Autodesk Inventor part; units mm, degrees
ref_plane "YZ Plane" through (0, 0, 0) normal (1, 0, 0) x (0, 1, 0)
ref_plane "XZ Plane" through (0, 0, 0) normal (0, 1, 0) x (-1, 0, 0)
ref_plane "XY Plane" through (0, 0, 0) normal (0, 0, 1) x (1, 0, 0)
sketch "Sketch1" plane through (0, 0, 0) normal (0, 0, 1) x (1, 0, 0)
  line L0 (-73, -33) -> (73, -33)
  line L1 (73, -33) -> (73, 33)
  line L2 (73, 33) -> (-73, 33)
  line L3 (-73, 33) -> (-73, -33)
  line L4 (-73, -33) -> (73, 33) construction
  line L5 (73, -33) -> (-73, 33) construction
  circle A0 centre (-20, 0) radius 9.5
  circle A1 centre (-50, 0) radius 9.5
  circle A2 centre (20, 0) radius 9.5
  circle A3 centre (50, 0) radius 9.5
  circle A4 centre (0, 0) radius 3.5
  dimension "d0" = 146
  dimension "d1" = 66
  dimension "d2" = 19
  dimension "d3" = 30
  dimension "d4" = 30
  dimension "d5" = 40
  dimension "d6" = 20
  dimension "d7" = 0
  dimension "d8" = 0
  dimension "d9" = 0
  dimension "d10" = 0
  dimension "d11" = 7
extrude "Extrusion1" add sketch "Sketch1" along normal blind 2
fillet "Fillet1" radius 2 4 edges at (0, -33, 2) (73, 0, 2) (0, 33, 2) (-73, 0, 2)
fillet "Fillet2" radius 2 4 edges at (-72.4142, -32.4142, 1.4142) (-72.4142, 32.4142, 1.4142) (72.4142, 32.4142, 1.4142) (72.4142, -32.4142, 1.4142)
equation "\"d4\" = d3"
properties part number "Cover"
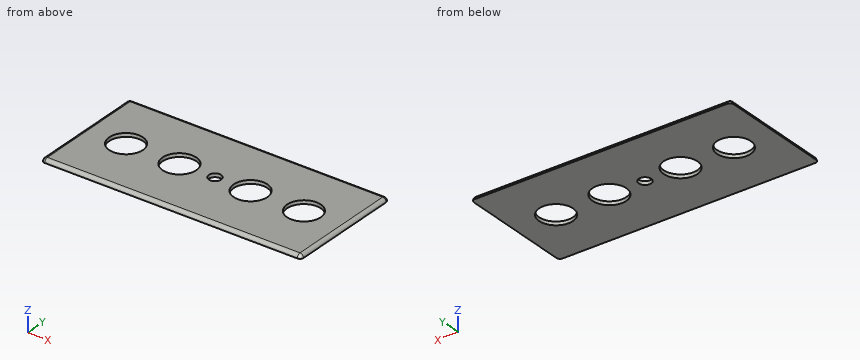
Here's how the part is built. I have some questions about the finished solid (model axes, mm). Coordinates: 2 decimals unless noted, no trailing zeros. Answer as a JSON object with one key per item and string values. Group by question number.
(1) Suppose I cut it at B-B, the plane y = 0. State how many separate pieces and enclosed holes the cut face has, then the cut area to 3 significant figures.
(2) I need wall thicknesses on probe 1 along X at (y, z) = (-8, 1.5); probe 2 along X at (y, z) = (-8.5, 0.85); probe 3 along Y at (x, z) = (20, 0.25). Which ranges of each line are inside material? Lowest first, please.
(3) For pin 1 (1 mm diameter, centred on x = 56, y = -6.5, fed in from -Z); pin 2 (1 mm diameter, centred on y = 20.5, z = 1, fed in from -X); pin 3 (1 mm diameter, centred on x = 44.5, z = 1, fed in from -Y); pin 4 (24.5 mm diameter, centred on x = -20, y = 0, fed in from +Z), each with a flat end and sliding along its axis, tell me the tip position at first contact or that it passes through.
Values found:
{
 "1": {"separate pieces": "6", "enclosed holes": "0", "area": "124 mm^2"},
 "2": {"probe 1": "x = -72.32 to -55.12, -44.88 to -25.12, -14.88 to 14.88, 25.12 to 44.88, 55.12 to 72.32", "probe 2": "x = -72.81 to -54.24, -45.76 to -24.24, -15.76 to 15.76, 24.24 to 45.76, 54.24 to 72.81", "probe 3": "y = -32.98 to -9.5, 9.5 to 32.98"},
 "3": {"pin 1": "passes through", "pin 2": "stops at x = -72.94", "pin 3": "stops at y = -32.94", "pin 4": "stops at z = 2"}
}
